Verification items for the finished model (mm, model axes). A direction names the side the tool comes from. Give positions to 0.01 mm unless a question says otherwise; leave off trailing zeros. Write each loop counter-clockwise with the first axis right and the second up, starting at its lowest first coordinate (ties: lowest second). Pieces come first, ordered by that corner, then holes. Notation, with made-up numbers: (58, -38.5) - (96, -38.5) arc R28 cw to (96, -2.5) - close; hole circle Ø9 at (45.25, 9.5). An arc over 180 degrees is marked (long way). Put each result on its own line as item: value.
Autodesk Inventor part; units mm, degrees
ref_plane "YZ Plane" through (0, 0, 0) normal (1, 0, 0) x (0, 1, 0)
ref_plane "XZ Plane" through (0, 0, 0) normal (0, 1, 0) x (-1, 0, 0)
ref_plane "XY Plane" through (0, 0, 0) normal (0, 0, 1) x (1, 0, 0)
sketch "Sketch1" plane through (0, 0, 0) normal (1, 0, 0) x (0, 1, 0)
  line L0 (0, 0) -> (1.65, 0) construction
  line L1 (1.65, 0) -> (3, 0) construction
  line L2 (4.9, 0) -> (4.9, -1.5)
  line L3 (4.9, -1.5) -> (3.9, -1.5)
  line L4 (3.9, -1.5) -> (3.9, -15)
  line L5 (3.9, -15) -> (1.7, -15)
  line L6 (1.7, -15) -> (1.7, -3)
  line L7 (0, 0) -> (0, -13.7466) construction
  line L8 (3, 0) -> (3, -3)
  line L9 (3, -3) -> (1.7, -3)
  line L10 (3, 0) -> (4.9, 0)
  dimension "d0" = 1.7
  dimension "d1" = 3.9
  dimension "d2" = 1
  dimension "d3" = 1.5
  dimension "d4" = 13.5
  dimension "d6" = 3
  dimension "d7" = 3
revolve "Revolution1" add sketch "Sketch1" angle 360 about axis through (0, 0, 0) along (0, 0, -1)
fillet "Fillet1" radius 0.5 2 edges at (0, -1.7, -15) (0, -3.9, -15)
sketch "Sketch2" plane through (0, 0, -3) normal (0, 0, 1) x (1, 0, 0)
  circle A0 centre (0, 0) radius 3
  line L0 (-1.7, 2.4718) -> (1.7, 2.4718) construction
  line L1 (1.7, 2.4718) -> (1.7, -2.4718)
  line L2 (1.7, -2.4718) -> (-1.7, -2.4718) construction
  line L3 (-1.7, -2.4718) -> (-1.7, 2.4718)
  circle A1 centre (0, 0) radius 1.7
  point P0 (-1.7, 0)
  point P1 (1.7, 0)
extrude "Extrusion1" cut sketch "Sketch2" against normal blind 0.2 contours L1 A1 L3 A0 | A0 L3 A1 L1
properties part number "HD_BearingShaft2"
Q1. Go/stop test with flat-tipped pins: pin 1 Ø0.9 at (x, y) = (-0.5, -2) entering from +Z; pin 2 Ø2 at (x, z) = (1.5, -11) entering from +Y; pin 3 Ø4 at (x, y) = (0, 0) entering from +Z; pin 4 Ø1.5 at (x, y) = (-0.5, 0) entering from +Z. Record where each tip stops, or that it passes through.
Answers follow:
pin 1: stops at z = -3.2
pin 2: stops at y = 3.87
pin 3: stops at z = -3
pin 4: passes through
Q2. Scan lines: line 1 along X through (y, z) = (0, -0.75); line 2 along X through (y, z) = (0, -1.75); line 3 along Z through (x, y) = (3.75, -2). Record each from-to range of solid material in increasing order.
Answers follow:
line 1: x = -4.9 to -3, 3 to 4.9
line 2: x = -3.9 to -3, 3 to 3.9
line 3: z = -1.5 to 0
Q3. Section check B-B, the plane z = -5.25. Record the cut outline in (x, y).
Answers follow:
outline: circle Ø7.8 at (0, 0); hole circle Ø3.4 at (0, 0)
Q4. Section check A-A, the plane x = 0. Record the cut outline in (y, z).
Answers follow:
outline: (-4.9, -1.5) - (-3.9, -1.5) - (-3.9, -14.5) arc R0.5 ccw to (-3.4, -15) - (-2.2, -15) arc R0.5 ccw to (-1.7, -14.5) - (-1.7, -3.2) - (-3, -3.2) - (-3, 0) - (-4.9, 0) - close; (1.7, -14.5) arc R0.5 ccw to (2.2, -15) - (3.4, -15) arc R0.5 ccw to (3.9, -14.5) - (3.9, -1.5) - (4.9, -1.5) - (4.9, 0) - (3, 0) - (3, -3.2) - (1.7, -3.2) - close
Q5. Release check for a two-part mould opening along Y. For faces 1 (the face through (0.513, 2.956, -1.622)), 2 (the face through (-4.783, -1.062, -0.76)), 3 (the face through (2, -2, -15)) record: released by +Y, released by -Y, zero draft, split by the parting line, or undercut.
Answers follow:
face 1: undercut
face 2: split by the parting line
face 3: zero draft
Q6. Set-up check for faces 4 (the face through (-1, -4, -1.5)), 5 (the face through (-3.2, -0.1, 0)), 6 (the face through (0, -2, -3.2)): record each of +Z, -Z, +X, -X, +Y, -Y from which the full face is reachable in a straight line by a thin tool's end or side.
Answers follow:
face 4: -Z
face 5: +Z, +X, -X, +Y, -Y
face 6: +Z
